Geometry check sheet. Reference: drawing and pictorial views, mm from the part's lowest x, y, z. A direction names the side the tool comes from. Round coordinates to 2 decimals unless told otherwise and drop trailing zeros. Write each loop counter-clockwise with the first axis right and the second up, starting at its lowest first coordinate (ties: lowest second). Pieces come first, ordered by that corner, then holes. Notation, with made-up numbers: M -36.75,-16.75 L -2.75,-16.75 A28 ccw -2.75,15.25 Z; hole C 22.5,30 d9. An arc over 180 degrees is marked long. Answer in a Markdown table with one row per item. Add a question column.
1. Set-up check for the marked faces 3, 4, 5, 6 and 7: record each of +Z, -Z, +X, -X, +Y, -Y from which the full face is reachable in a straight line by a thin tool's end or side.
2. Go/stop test with flat-tipped pins: pin 1 Ø1 at (x, y) = (24.5, 1.5) entering from +Z; pin 2 Ø2 at (y, z) = (7.5, 8.5) entering from +X; pin 3 Ø1.8 at (y, z) = (2.5, 12) entering from +X. Record where each tip stops, or that it passes through.
3. Sectioned sample at D-D on y = 2.25. Count the separate pieces of the cut face and the enclosed holes in it, plus the area to 3 significant figures.
4. Sectioned sample at A-A on x = 9.25. Record the cut outline in (y, z).
5. Draft check along X on the marked faces 1 and 2. Enter one of: pulls with the +X half, pulls with the -X half, needs draft (parallel to the pull), parting line crosses it, or undercut.
6. Sectioned sample at B-B on y = 6.75. Record the cut outline in (x, z), plus the area to 3 significant figures.
7. Sectioned sample at C-C on z = 10. Record the cut outline in (x, y).
8. Material ranges on probe 1 along X at (y, z) = (7.5, 9.75); probe 2 along Z at (x, y) = (36.5, 2.25) (1 decimal); probe 3 along Y at (x, z) = (15.5, 10.25), recorded low to high.
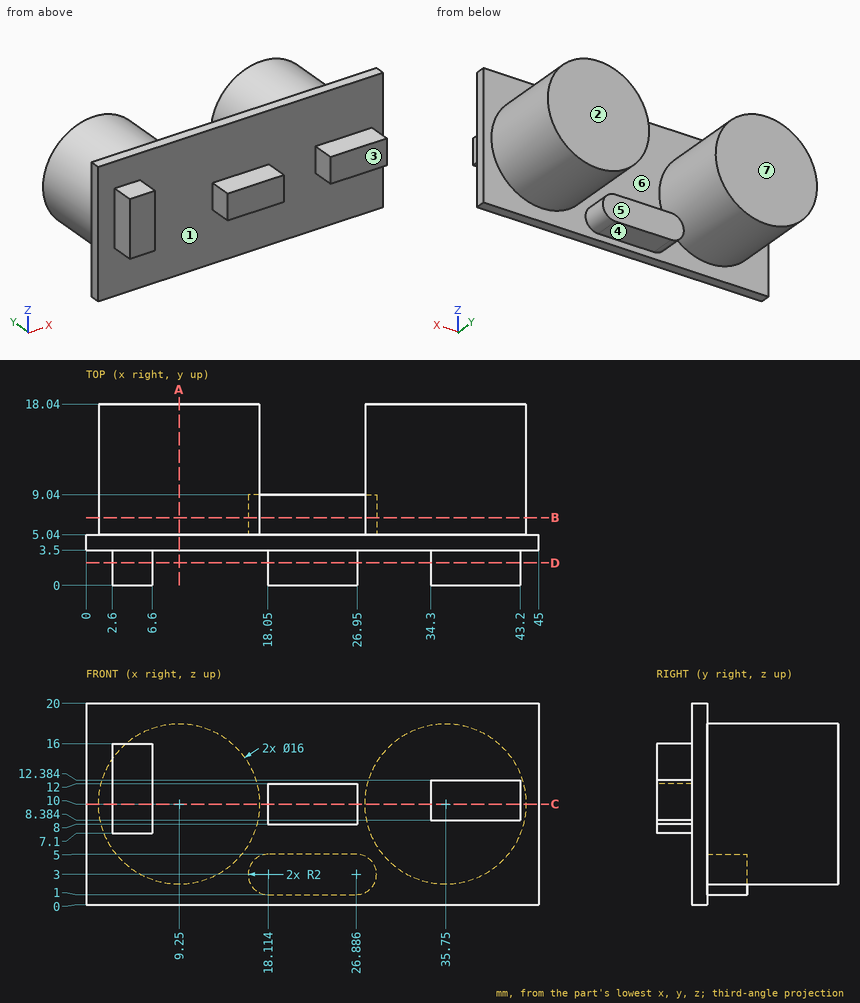
Geometry check:
| question | item | result |
|---|---|---|
| 1 | face 3 | +Z, -Z, +X, -X, -Y |
| 1 | face 4 | -Z, +X, -X, +Y |
| 1 | face 5 | -Z, +Y |
| 1 | face 6 | +Y |
| 1 | face 7 | +Z, -Z, +X, -X, +Y |
| 2 | pin 1 | stops at z = 12 |
| 2 | pin 2 | stops at x = 43.73 |
| 2 | pin 3 | stops at x = 43.2 |
| 3 | separate pieces | 3 |
| 3 | enclosed holes | 0 |
| 3 | area | 107 mm2 |
| 4 | outline | M 3.5,0 L 5.04,0 L 5.04,2 L 18.04,2 L 18.04,18 L 5.04,18 L 5.04,20 L 3.5,20 Z |
| 5 | face 1 | undercut |
| 5 | face 2 | needs draft |
| 6 | outline | C 9.25,10 d16; M 18.11,1 L 26.89,1 A2 ccw 26.89,5 L 18.11,5 A2 ccw Z; C 35.75,10 d16 |
| 6 | area | 450 mm2 |
| 7 | outline | M 0,3.5 L 2.6,3.5 L 2.6,0 L 6.6,0 L 6.6,3.5 L 18.05,3.5 L 18.05,0 L 26.95,0 L 26.95,3.5 L 34.3,3.5 L 34.3,0 L 43.2,0 L 43.2,3.5 L 45,3.5 L 45,5.04 L 43.75,5.04 L 43.75,18.04 L 27.75,18.04 L 27.75,5.04 L 17.25,5.04 L 17.25,18.04 L 1.25,18.04 L 1.25,5.04 L 0,5.04 Z |
| 8 | probe 1 | x = 1.25 to 17.25, 27.75 to 43.75 |
| 8 | probe 2 | z = 8.4 to 12.4 |
| 8 | probe 3 | y = 3.5 to 18.04 |
